Geometry: final body of the model. Coordinates: model frame, mm. Face numbers are marked on the shaded views. Coordinates: 2 decimals unless noted, no trailing zeros. Order: outer loops, then holes, each group sorted by start corner. A loop starts at its lowest first (then second) coordinate and runs counter-clockwise, first axis right, second up. Notation, with made-up numbers: (51, 60.5) -> (79, 60.5) arc R18 ccw to (79, 72.5) -> close; hole circle Ø7 at (2, -30). An arc over 180 degrees is marked (long way). Answer in a Markdown table with one row per item. Add a question column.
1) Pull-direction query (Y, two-part tool) for the marked faces 1, 2, 3 and 4; classes: +Y half, -Y half, draft (parallel to the pull), parting line (faces both ways), or undercut.
2) Section query C-C on x = -6. Return the cut outline in (y, z) (3 decimals), then the cut area to 3 significant figures.
3) Ray query, line 1 (X direction, y = 5, z = 1.65) (3 decimals); line 2 (Y direction, x = -15.5, z = 1.85) (3 decimals); line 3 (X direction, y = 8.5, z = 0.2). Return the intervals inside material, ascending. Write a range as from..to.
4) Section query D-D on y = 5. Count the separate pieces of the cut face and the enclosed holes in it, then the cut area to 4 significant figures.
5) Section query B-B on z = 1.2. Return the cut outline in (x, y) (3 decimals), then the cut area to 3 significant figures.
6) Section query A-A on x = -44. Return the cut outline in (y, z).
7) Contact query for flat-ended pins moving along their axis: P1, Ø4.5, axis at x = -5.5, y = 6, coming from the -Z side; P2, Ø4.5, axis at x = -16, y = 3.5, coming from the -Z side. Output: stop coordinate, or through.
```python
from build123d import *

# Parameters (mm, degrees)
SKETCH_1_W          = 50
SKETCH_1_H          = 10
EXTRUDE_1_DEPTH     = 3
SKETCH_1_3_R        = 3.7
SKETCH_1_3_R_2      = 3.675
SKETCH_1_3_R_3      = 3.65
SKETCH_1_3_R_4      = 3.6
SKETCH_1_3_R_5      = 3.625
CUT_EXTRUDE_1_DEPTH = 4
SKETCH_1_4_R        = 4.3
SKETCH_1_4_R_2      = 3.7
SKETCH_1_4_R_3      = 4.35
SKETCH_1_4_R_4      = 3.65
SKETCH_1_4_R_5      = 4.325
SKETCH_1_4_R_6      = 3.675
SKETCH_1_4_R_7      = 3.625
SKETCH_1_4_R_8      = 3.6
CUT_EXTRUDE_2_DEPTH = 0.6
FILLET_4_R          = 3


with BuildPart() as part:
    # Sketch 1 → Extrude 1 (new body)
    with BuildSketch(Plane.XY):
        with Locations((-25, 5)):
            Rectangle(SKETCH_1_W, SKETCH_1_H)
    extrude(amount=EXTRUDE_1_DEPTH)

    # Sketch 1_3 → Cut-Extrude 1 (cut, through all)
    with BuildSketch(Plane.XY):
        with Locations((-25, 5)):
            Circle(SKETCH_1_3_R)
        with Locations((-34.5, 5)):
            Circle(SKETCH_1_3_R_2)
        with Locations((-44, 5)):
            Circle(SKETCH_1_3_R_3)
        with Locations((-6, 5)):
            Circle(SKETCH_1_3_R_4)
        with Locations((-15.5, 5)):
            Circle(SKETCH_1_3_R_5)
    extrude(amount=CUT_EXTRUDE_1_DEPTH, mode=Mode.SUBTRACT)

    # Sketch 1_4 → Cut-Extrude 2 (cut)
    with BuildSketch(Plane.XY):
        with Locations((-25, 5)):
            Circle(SKETCH_1_4_R)
        with Locations((-25, 5)):
            Circle(SKETCH_1_4_R_2, mode=Mode.SUBTRACT)
        with Locations((-44, 5)):
            Circle(SKETCH_1_4_R_3)
        with Locations((-44, 5)):
            Circle(SKETCH_1_4_R_4, mode=Mode.SUBTRACT)
        with Locations((-34.5, 5)):
            Circle(SKETCH_1_4_R_5)
        with Locations((-34.5, 5)):
            Circle(SKETCH_1_4_R_6, mode=Mode.SUBTRACT)
        with Locations((-15.5, 5)):
            Circle(SKETCH_1_4_R_5)
        with Locations((-15.5, 5)):
            Circle(SKETCH_1_4_R_7, mode=Mode.SUBTRACT)
        with Locations((-6, 5)):
            Circle(SKETCH_1_4_R_5)
        with Locations((-6, 5)):
            Circle(SKETCH_1_4_R_8, mode=Mode.SUBTRACT)
    extrude(amount=CUT_EXTRUDE_2_DEPTH, mode=Mode.SUBTRACT)

    # Fillet 4
    fillet_4_edges = [part.edges().sort_by_distance(p)[0] for p in [
        (-50, 10, 1.5),
        (0, 10, 1.5),
        (0, 0, 1.5),
        (-50, 0, 1.5),
    ]]
    fillet(fillet_4_edges, radius=FILLET_4_R)


solid = part.part
```
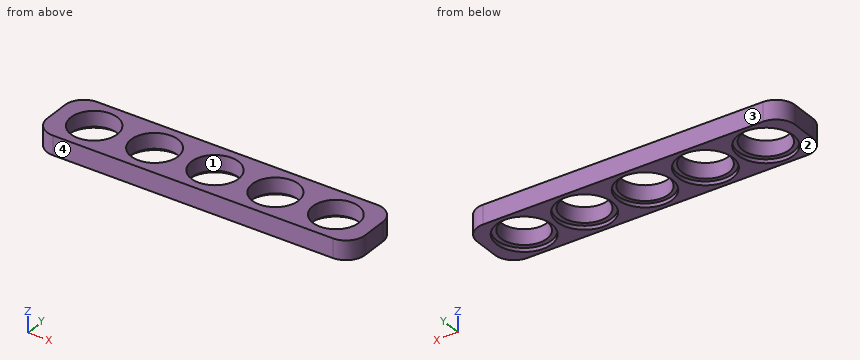
Result:
| question | item | result |
|---|---|---|
| 1 | face 1 | undercut |
| 1 | face 2 | draft |
| 1 | face 3 | +Y half |
| 1 | face 4 | -Y half |
| 2 | outline | (0, 0) -> (0.675, 0) -> (0.675, 0.6) -> (1.4, 0.6) -> (1.4, 3) -> (0, 3) -> close; (8.6, 0.6) -> (9.325, 0.6) -> (9.325, 0) -> (10, 0) -> (10, 3) -> (8.6, 3) -> close |
| 2 | area | 7.53 mm2 |
| 3 | line 1 | -50..-47.65, -40.35..-38.175, -30.825..-28.7, -21.3..-19.125, -11.875..-9.6, -2.4..0 |
| 3 | line 2 | 0..1.375, 8.625..10 |
| 3 | line 3 | -49.6..-46.58, -41.42..-37.04, -31.96..-27.5, -22.5..-18.04, -12.96..-8.54, -3.46..-0.4 |
| 4 | separate pieces | 6 |
| 4 | enclosed holes | 0 |
| 4 | area | 36.45 mm2 |
| 5 | outline | (-50, 3) arc R3 ccw to (-47, 0) -> (-3, 0) arc R3 ccw to (0, 3) -> (0, 7) arc R3 ccw to (-3, 10) -> (-47, 10) arc R3 ccw to (-50, 7) -> close; hole circle Ø7.3 at (-44, 5); hole circle Ø7.35 at (-34.5, 5); hole circle Ø7.4 at (-25, 5); hole circle Ø7.25 at (-15.5, 5); hole circle Ø7.2 at (-6, 5) |
| 5 | area | 283 mm2 |
| 6 | outline | (0, 0) -> (0.65, 0) -> (0.65, 0.6) -> (1.35, 0.6) -> (1.35, 3) -> (0, 3) -> close; (8.65, 0.6) -> (9.35, 0.6) -> (9.35, 0) -> (10, 0) -> (10, 3) -> (8.65, 3) -> close |
| 7 | P1 | through |
| 7 | P2 | z = 0.6 |
